```python
from build123d import *

# Parameters (mm, degrees)
F1_DEPTH = 138.176
F2_E3_W  = 14.2383185016
F2_E3_H  = 142.748
F3_DEPTH = 3.556
F4_E2_W  = 109.4098263908
F4_E2_H  = 141.224
F5_DEPTH = 3.556


with BuildPart() as f1:
    # F0 (on Right) → F1 (new body)
    with BuildSketch(Plane.YZ):
        Polygon((51.4731071889, 72.4924988879), (-41.5385216475, 55.4317318249), (-41.5385216475, -3.5118000333), (51.4731071889, -4.5339060016), align=None)
    extrude(amount=F1_DEPTH)

    # F2_E3 (on explicit) → F3 (join)
    with BuildSketch(Plane(origin=(0, -41.5385216475, 55.4317318249), x_dir=(0, -0.9835903566, -0.1804162143), z_dir=(0, -0.1804162143, 0.9835903566))):
        with Locations((7.1191592508, 71.374)):
            Rectangle(F2_E3_W, F2_E3_H)
    extrude(amount=-F3_DEPTH)

    # F4_E2 (on explicit) → F5 (join)
    with BuildSketch(Plane(origin=(0, 66.0759285092, 75.1710385084), x_dir=(0, -0.9835903566, -0.1804162143), z_dir=(0, -0.1804162143, 0.9835903566))):
        with Locations((54.7049131954, 70.612)):
            Rectangle(F4_E2_W, F4_E2_H)
    extrude(amount=-F5_DEPTH)


solid = f1.part
```
Here's how the part is built. I have some questions about the finished solid (model axes, mm). Round coordinates to 2 decimals unless told otherwise and drop trailing zeros. Order: outer loops, then holes, each group sorted by start corner. A loop starts at its lowest first (then second) coordinate and runs counter-clockwise, first axis right, second up. Notation, with made-up numbers: (78.5, 64) -> (127.5, 64) arc R17 cw to (127.5, 93) -> close; hole circle Ø11 at (86.25, 27). An arc over 180 degrees is marked (long way). Use a Markdown table: item, result. Add a question column.
(1) For pin 1 Ø8 at (y, z) = (-26.5, 5.5) entering from +X; pin 2 Ø6 at (x, z) = (92, 37) entering from +Y; pin 3 Ø5 at (y, z) = (-8.5, 10) entering from -X; pin 4 Ø2 at (x, y) = (114.5, -27) entering from +Z, each with a flat end and sliding along its axis, tell me the tip position at first contact or that it passes through.
(2) I need wall thicknesses on line 1 along Y through (x, z) = (26.5, 20); line 2 along X through (y, z) = (-41, 47); line 3 along X through (y, z) = (-26, 56). Which ranges of each line are inside material? Lowest first, please.
(3) If we mould it in two halves opening along Y, with no side actions, what happens to faces 1 (the face through (82.28, 55.74, 69.66)), 2 (the face through (70.375, -55.227, 51.139)), 3 (the face through (141.224, 13, 64)), 4 (the face through (68, 51.473, 32))? For each: released by +Y, released by -Y, zero draft, split by the parting line, or undercut.
(4) Suppose I cut it at D-D, the plane y = -30. Please give me the cut outline in (x, z), and give its area (3 significant figures).
(5) Suppose I cut it at A-A, the plane x = 125.5. Please give me the cut outline in (y, z).
(6) Suppose I cut it at B-B, the plane y = 28. Please give me the cut outline in (x, z), and give its area (3 significant figures).
(7) Suppose I cut it at C-C, the plane z = 12.5. Please give me the cut outline in (x, y).
Verdict:
| question | item | result |
|---|---|---|
| 1 | pin 1 | x = 138.18 |
| 1 | pin 2 | y = 51.47 |
| 1 | pin 3 | x = 0 |
| 1 | pin 4 | z = 58.28 |
| 2 | line 1 | -41.54 to 51.47 |
| 2 | line 2 | 0 to 138.18 |
| 2 | line 3 | 0 to 141.22 |
| 3 | face 1 | undercut |
| 3 | face 2 | released by -Y |
| 3 | face 3 | zero draft |
| 3 | face 4 | released by +Y |
| 4 | outline | (0, -3.64) -> (138.18, -3.64) -> (138.18, 53.93) -> (141.22, 53.93) -> (141.22, 57.55) -> (0, 57.55) -> close |
| 4 | area | 8,470 mm2 |
| 5 | outline | (-55.54, 52.86) -> (-54.9, 49.37) -> (-41.54, 51.82) -> (-41.54, -3.51) -> (51.47, -4.53) -> (51.47, 68.88) -> (66.72, 71.67) -> (66.08, 75.17) -> close |
| 6 | outline | (0, -4.28) -> (138.18, -4.28) -> (138.18, 64.57) -> (141.22, 64.57) -> (141.22, 68.19) -> (0, 68.19) -> close |
| 6 | area | 10,000 mm2 |
| 7 | outline | (0, -41.54) -> (138.18, -41.54) -> (138.18, 51.47) -> (0, 51.47) -> close |
